Read the model definition and answer for the solid it produces. Units are mm, in the model's axes. A direction names the side the tool comes from. Coordinates: 2 decimals unless noted, no trailing zeros. Write each loop counter-clockwise with the first axis right and the second up, starting at its lowest first coordinate (ties: lowest second). Pieces come first, ordered by that corner, then holes.
1) The part is cut by section D-D (x = 4.95). Determine the outline of the cut face in (y, z) (3 decimals).
2) Which of the six approach directions +Z, -Z, +X, -X, +Y, -Y give full straight-line access (tool end or side, diameter ignored) to faces 4 (the face through (-2, 2, 23)), 5 (the face through (0, 2, 32.5))?
3) The part is cut by section A-A (z = -4). Determine the outline of the cut face in (x, y) (3 decimals), then the cut area to 4 significant figures.
4) This flat-tipped pin is pushed along its axis until it touches: pin 1 Ø3 at (x, z) = (-4.95, -24) entering from -Y. Where does it stop, or does it pass through?
5) Determine the mould class of faces 1 (the face through (16, 2, 31)), 2 (the face through (0, 2, -32.5)), 3 (the face through (14, 3.175, 0)) for opening direction Z: +Z half, -Z half, draft (parallel to the pull), parting line (faces both ways), or undercut.
6) The part is cut by section B-B (x = 0). Determine the outline of the cut face in (y, z) (3 decimals).
7) Find the intervals of material crossed by line 1 (X direction, y = 0.9, z = -24); line 2 (X direction, y = 2.45, z = 24); line 3 (Z direction, x = -7, y = 1.25), in increasing order.
8) The part is cut by section C-C (z = 8). Determine the outline of the cut face in (x, y) (3 decimals), then the cut area to 4 significant figures.
from build123d import *

# Parameters (mm, degrees)
SKETCH1_W           = 43
SKETCH1_H           = 65
SKETCH1_R           = 1.65
BOSS_EXTRUDE1_DEPTH = 3.175
CUT_EXTRUDE1_DEPTH  = 3.175


with BuildPart() as part:
    # Sketch1 → Boss-Extrude1 (new body)
    with BuildSketch(Plane(origin=(0, 0, 0), x_dir=(1, 0, 0), z_dir=(0, 1, 0))):
        Rectangle(SKETCH1_W, SKETCH1_H)
        with Locations(Location((-4.95, -24, 0), (0, 0, 270))):
            Circle(SKETCH1_R, mode=Mode.SUBTRACT)
        with BuildLine():
            Line((-10.5, 21), (-2, 21))
            Line((-2, 21), (-2, 24))
            Line((-2, 24), (-2, 25))
            ThreePointArc((-2, 25), (0, 27), (2, 25))
            Line((2, 25), (2, 24))
            Line((2, 24), (2, 21))
            Line((2, 21), (10.5, 21))
            Line((10.5, 21), (10.5, 0))
            Line((10.5, 0), (10.5, -21))
            Line((10.5, -21), (2, -21))
            Line((2, -21), (2, -24))
            Line((2, -24), (2, -25))
            ThreePointArc((2, -25), (0, -27), (-2, -25))
            Line((-2, -25), (-2, -24))
            Line((-2, -24), (-2, -21))
            Line((-2, -21), (-10.5, -21))
            Line((-10.5, -21), (-10.5, 0))
            Line((-10.5, 0), (-10.5, 21))
        make_face(mode=Mode.SUBTRACT)
        with BuildLine():
            ThreePointArc((6.6, -24), (4.95, -25.65), (3.3, -24))
            ThreePointArc((3.3, -24), (4.95, -22.35), (6.6, -24))
        make_face(mode=Mode.SUBTRACT)
        with Locations(Location((-4.95, 24, 0), (0, 0, 270))):
            Circle(SKETCH1_R, mode=Mode.SUBTRACT)
        with BuildLine():
            ThreePointArc((6.6, 24), (4.95, 22.35), (3.3, 24))
            ThreePointArc((3.3, 24), (4.95, 25.65), (6.6, 24))
        make_face(mode=Mode.SUBTRACT)
    extrude(amount=BOSS_EXTRUDE1_DEPTH)

    # Sketch3 → Cut-Extrude1 (cut)
    with BuildSketch(Plane(origin=(0, 3.175, 0), x_dir=(1, 0, 0), z_dir=(0, 1, 0))):
        with BuildLine():
            Line((-14, -21), (-14, -29))
            ThreePointArc((-14, -29), (-16, -31), (-18, -29))
            Line((-18, -29), (-18, -21))
            ThreePointArc((-18, -21), (-16, -19), (-14, -21))
        make_face()
        with BuildLine():
            Line((14, -21), (14, -29))
            ThreePointArc((14, -29), (16, -31), (18, -29))
            Line((18, -29), (18, -21))
            ThreePointArc((18, -21), (16, -19), (14, -21))
        make_face()
        with BuildLine():
            Line((-14, 11), (-14, 3))
            ThreePointArc((-14, 3), (-16, 1), (-18, 3))
            Line((-18, 3), (-18, 11))
            ThreePointArc((-18, 11), (-16, 13), (-14, 11))
        make_face()
        with BuildLine():
            Line((14, 11), (14, 3))
            ThreePointArc((14, 3), (16, 1), (18, 3))
            Line((18, 3), (18, 11))
            ThreePointArc((18, 11), (16, 13), (14, 11))
        make_face()
    extrude(amount=-CUT_EXTRUDE1_DEPTH, mode=Mode.SUBTRACT)


solid = part.part
Reported:
1. outline: (0, -32.5) - (3.175, -32.5) - (3.175, -25.65) - (0, -25.65) - close; (0, -22.35) - (3.175, -22.35) - (3.175, -21) - (0, -21) - close; (0, 21) - (3.175, 21) - (3.175, 22.35) - (0, 22.35) - close; (0, 25.65) - (3.175, 25.65) - (3.175, 32.5) - (0, 32.5) - close
2. face 4: +Y, -Y
2. face 5: +Z, +X, -X, +Y, -Y
3. outline: (-21.5, 0) - (-18, 0) - (-18, 3.175) - (-21.5, 3.175) - close; (-14, 0) - (-10.5, 0) - (-10.5, 3.175) - (-14, 3.175) - close; (10.5, 0) - (14, 0) - (14, 3.175) - (10.5, 3.175) - close; (18, 0) - (21.5, 0) - (21.5, 3.175) - (18, 3.175) - close
3. area: 44.45 mm2
4. pin 1: passes through
5. face 1: undercut
5. face 2: -Z half
5. face 3: draft
6. outline: (0, -32.5) - (3.175, -32.5) - (3.175, -27) - (0, -27) - close; (0, 27) - (3.175, 27) - (3.175, 32.5) - (0, 32.5) - close
7. line 1: x = -21.5 to -6.6, -3.3 to -2, 2 to 3.3, 6.6 to 21.5
7. line 2: x = -21.5 to -18, -14 to -6.6, -3.3 to -2, 2 to 3.3, 6.6 to 14, 18 to 21.5
7. line 3: z = -32.5 to -21, 21 to 32.5
8. outline: (-21.5, 0) - (-10.5, 0) - (-10.5, 3.175) - (-21.5, 3.175) - close; (10.5, 0) - (21.5, 0) - (21.5, 3.175) - (10.5, 3.175) - close
8. area: 69.85 mm2
